```python
from build123d import *

# Parameters (mm, degrees)
ESQUISSE2_OUTSIDE_W     = 12.304
ESQUISSE2_OUTSIDE_H     = 12.304
ENL_V_MAT_EXTRU_1_DEPTH = 3.924186047


with BuildPart() as part:
    # Esquisse1 → Base-Révolution (revolve)
    with BuildSketch(Plane.XY, mode=Mode.PRIVATE) as base_r_volution_sk:
        with BuildLine():
            Line((-0.531153927, 0), (-2.75, 0))
            Line((-2.75, 0), (-2.75, 4))
            Line((-2.75, 4), (-3.352191691, 4))
            Line((-3.352191691, 4), (-3.352191691, 7))
            Line((-3.352191691, 7), (-3, 7))
            Line((-3, 7), (-3, 10.543617096))
            Line((-3, 10.543617096), (-2.340835241, 10.924186047))
            Line((-2.340835241, 10.924186047), (-0.5, 10.924186047))
            Line((-0.5, 10.924186047), (-0.5, 14))
            ThreePointArc((-0.5, 14), (-0.353553391, 14.353553391), (0, 14.5))
            Line((0, 14.5), (0, -0.8))
            Line((0, -0.8), (-0.531153927, 0))
        make_face()
    revolve(base_r_volution_sk.sketch.rotate(Axis((0, 14.968764899, 0), (0, -1, 0)), 270), axis=Axis((0, 14.968764899, 0), (0, -1, 0)))

    # Esquisse2 outside → Enlèv. mat.-Extru.1 (cut)
    with BuildSketch(Plane(origin=(0, 10.924186047, 0), x_dir=(-1, 0, 0), z_dir=(0, 1, 0))):
        Rectangle(ESQUISSE2_OUTSIDE_W, ESQUISSE2_OUTSIDE_H)
        Polygon((0, 2.886751346), (-2.5, 1.443375673), (-2.5, -1.443375673), (0, -2.886751346), (2.5, -1.443375673), (2.5, 1.443375673), align=None, mode=Mode.SUBTRACT)
    extrude(amount=-ENL_V_MAT_EXTRU_1_DEPTH, mode=Mode.SUBTRACT)


solid = part.part
```
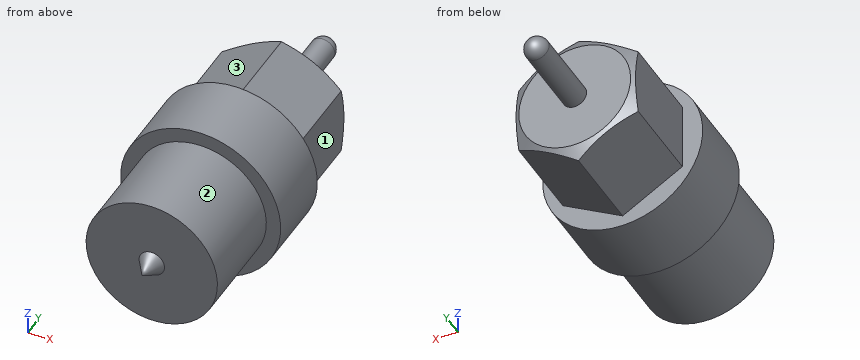
CAD build for the part. Positions are in the model's coordinates, mm. Face numbers are marked on the shaded views. A direction names the side the tool comes from. Coordinates: 2 decimals unless noted, no trailing zeros. Write each loop counter-clockwise with the first axis right and the second up, starting at its lowest first coordinate (ties: lowest second). Pieces come first, ordered by that corner, then holes.
(1) Cut at C-C, the plane x = -3. List the corners of the cut face in (y, z).
(2) Cut at B-B, the plane y = 3.75. List the corners of the cut face in (x, z).
(3) Drill centre lines: probe 1 along Y at (x, z) = (2, 0.5); probe 2 along Y at (x, z) = (2, -2.5); probe 3 along X at (y, z) = (2, 0). Where is each one in solid material? Low to high.
(4) 3-axis set-ups, long thin cutter, end or side, ignore diameter. For the marked faces 1, 2 and 3: which of +Z, -Z, +X, -X, +Y, -Y reach the whole face in a straight line?
(5) Flat gauge pins, fed straight in: pin 1 (1.4 mm diameter, centred on y = 9, z = 0.5, fed in from -X); pin 2 (0.9 mm diameter, centred on y = 8.5, z = 0, fed in from +X); pin 3 (1 mm diameter, centred on x = 0.5, z = -2, fed in from +Y). Where does each tip first touch, or does it go through?
(6) Cut at D-D, the plane y = 11.75. List the corners of the cut face in (x, z), and give its area (3 significant figures).
(7) Cut at A-A, the plane y = 7.75. List the corners of the cut face in (x, z).
Geometry says:
1. outline: (4, -1.5) - (7, -1.5) - (7, 1.5) - (4, 1.5) - close
2. outline: circle Ø5.5 at (0, 0)
3. probe 1: y = 0 to 10.92
3. probe 2: y = 4 to 7
3. probe 3: x = -2.75 to 2.75
4. face 1: +Z, -Z, +X, +Y
4. face 2: -Y
4. face 3: +Z, -X, +Y
5. pin 1: stops at x = -2.5
5. pin 2: stops at x = 2.5
5. pin 3: stops at y = 10.92
6. outline: circle Ø1 at (0, 0)
6. area: 0.785 mm2
7. outline: (-2.5, -1.44) - (0, -2.89) - (2.5, -1.44) - (2.5, 1.44) - (0, 2.89) - (-2.5, 1.44) - close
